```python
from build123d import *

# Parameters (mm, degrees)
F1_DEPTH = 50.8
F3_DEPTH = 50.801
F4_R     = 9.525
F5_DEPTH = 50.801
F6_R     = 63.5
F6_W     = 50.8
F6_H     = 50.8
F7_DEPTH = 12.7
F8_R     = 3.81


with BuildPart() as f1:
    # F0 (on Front) → F1 (new body)
    with BuildSketch(Plane.XZ):
        Polygon((-38.3064501607, 0), (-38.3064501607, 59.24468064), (-51.0064501607, 59.24468064), (-51.0064501607, -16.95531936), (-0.2064501607, -16.95531936), (-0.2064501607, 59.24468064), (-12.9064501607, 59.24468064), (-12.9064501607, 0), align=None)
    extrude(amount=F1_DEPTH)

    # F2 (on face) → F3 (cut, through all)
    with BuildSketch(Plane.YZ.offset(-0.2064501607)):
        with BuildLine():
            ThreePointArc((-50.8, 33.84468064), (-43.3605122421, 51.8051928821), (-25.4, 59.24468064))
            Line((-25.4, 59.24468064), (-50.8, 59.24468064))
            Line((-50.8, 59.24468064), (-50.8, 33.84468064))
        make_face()
        with BuildLine():
            ThreePointArc((-25.4, 59.24468064), (-7.4394877579, 51.8051928821), (0, 33.84468064))
            Line((0, 33.84468064), (0, 59.24468064))
            Line((0, 59.24468064), (-25.4, 59.24468064))
        make_face()
    extrude(amount=-F3_DEPTH, mode=Mode.SUBTRACT)

    # F4 (on face) → F5 (cut, through all)
    with BuildSketch(Plane.YZ.offset(-0.2064501607)):
        with Locations((-25.4, 33.84468064)):
            Circle(F4_R)
    extrude(amount=-F5_DEPTH, mode=Mode.SUBTRACT)

    # F6 (on face) → F7 (join)
    with BuildSketch(Plane(origin=(0, 0, -16.95531936), x_dir=(1, 0, 0), z_dir=(0, 0, -1))):
        with Locations((-25.6064501607, 25.4)):
            Circle(F6_R)
        with BuildLine():
            ThreePointArc((-19.2726698552, 69.3964285714), (5.824446263, 56.8308964237), (18.3899784107, 31.7337803056))
            ThreePointArc((18.3899784107, 31.7337803056), (23.1703455028, 30.0477240974), (25.1935498393, 25.4))
            ThreePointArc((25.1935498393, 25.4), (23.1703455028, 20.7522759026), (18.3899784107, 19.0662196944))
            ThreePointArc((18.3899784107, 19.0662196944), (5.824446263, -6.0308964237), (-19.2726698552, -18.5964285714))
            ThreePointArc((-19.2726698552, -18.5964285714), (-19.2605063799, -18.8230693282), (-19.2564501607, -19.05))
            ThreePointArc((-19.2564501607, -19.05), (-25.8333808326, -25.3959437809), (-31.9402304663, -18.5964285714))
            ThreePointArc((-31.9402304663, -18.5964285714), (-57.0373465845, -6.0308964237), (-69.6028787322, 19.0662196944))
            ThreePointArc((-69.6028787322, 19.0662196944), (-76.4064501607, 25.4), (-69.6028787322, 31.7337803056))
            ThreePointArc((-69.6028787322, 31.7337803056), (-57.0373465845, 56.8308964237), (-31.9402304663, 69.3964285714))
            ThreePointArc((-31.9402304663, 69.3964285714), (-25.8333808326, 76.1959437809), (-19.2564501607, 69.85))
            ThreePointArc((-19.2564501607, 69.85), (-19.2605063799, 69.6230693282), (-19.2726698552, 69.3964285714))
        make_face(mode=Mode.SUBTRACT)
        with BuildLine():
            ThreePointArc((18.3899784107, 19.0662196944), (12.4935498393, 25.4), (18.3899784107, 31.7337803056))
            ThreePointArc((18.3899784107, 31.7337803056), (5.824446263, 56.8308964237), (-19.2726698552, 69.3964285714))
            ThreePointArc((-19.2726698552, 69.3964285714), (-25.6064501607, 63.5), (-31.9402304663, 69.3964285714))
            ThreePointArc((-31.9402304663, 69.3964285714), (-57.0373465845, 56.8308964237), (-69.6028787322, 31.7337803056))
            ThreePointArc((-69.6028787322, 31.7337803056), (-65.4087260633, 29.7267956636), (-63.7064501607, 25.4))
            ThreePointArc((-63.7064501607, 25.4), (-65.4087260633, 21.0732043364), (-69.6028787322, 19.0662196944))
            ThreePointArc((-69.6028787322, 19.0662196944), (-57.0373465845, -6.0308964237), (-31.9402304663, -18.5964285714))
            ThreePointArc((-31.9402304663, -18.5964285714), (-25.6064501607, -12.7), (-19.2726698552, -18.5964285714))
            ThreePointArc((-19.2726698552, -18.5964285714), (5.824446263, -6.0308964237), (18.3899784107, 19.0662196944))
        make_face()
        with Locations((-25.6064501607, 25.4)):
            Rectangle(F6_W, F6_H, mode=Mode.SUBTRACT)
        with Locations((-25.6064501607, 25.4)):
            Rectangle(F6_W, F6_H)
    extrude(amount=F7_DEPTH)

    # F8
    f8_edges = [f1.edges().sort_by_distance(p)[0] for p in [
        (-51.00645, -25.4, -16.955319),
        (-25.60645, -50.8, -16.955319),
        (-0.20645, -25.4, -16.955319),
        (-25.60645, 0, -16.955319),
        (-89.10645, -25.4, -16.955319),
    ]]
    fillet(f8_edges, radius=F8_R)


solid = f1.part
```
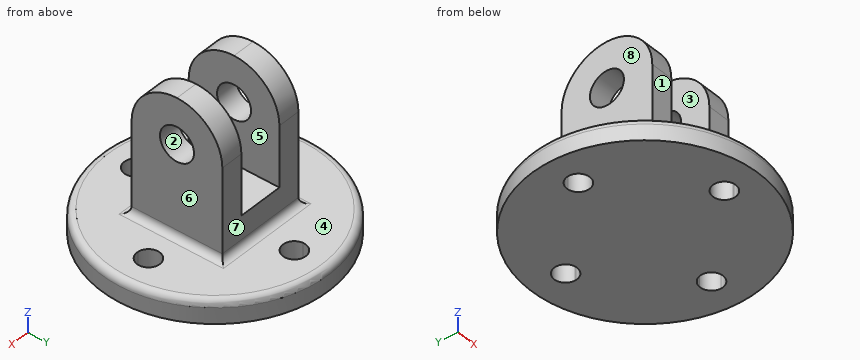
CAD build for the part. Positions are in the model's coordinates, mm. Face numbers are marked on the shaded views. A direction names the side the tool comes from. Round coordinates to 2 decimals unless told otherwise and drop trailing zeros. Order: outer loops, then holes, each group sorted by start corner. A loop starts at its lowest first (then second) coordinate and runs counter-clockwise, first axis right, second up. Notation, with made-up numbers: (16.25, 46.25) - (23.25, 46.25) arc R24 cw to (23.25, 82.25) - close; hole circle Ø3 at (68, 10.5). An arc over 180 degrees is marked (long way). Use CSV: the item, a comma, the result in double quotes. Start each with the question number.
1) Wall check: L1, parallel to X at y = -40.5, z = 44; L2, parallel to Z at x = -8, y = -25; L3, parallel to Y at x = -40, z = 29. Give the ranges that are in metal, low to high. Write a range as [from, to].
2) Saw through at B-B (z = 18). List the corners of the cut face in (x, y), and give its area (3 significant figures).
3) Pin check, flat tips, straight feed: pin 1 Ø5 at (y, z) = (-9, 35) entering from +X; pin 2 Ø14 at (x, z) = (-36, 18.5) entering from -Y; pin 3 Ø3 at (x, z) = (-41, 48.5) entering from +Y. Stop position of each tip, or through.
4) Saw through at A-A (z = -23). List the corners of the cut face in (x, y).
5) Saw through at C-C (z = -7). List the corners of the cut face in (x, y).
6) Tool access for the marked faces 4, 5, 6, 7 and 8: list every direction of +Z, -Z, +X, -X, +Y, -Y with a clear straight run to the whole face (end or side of a thin tool).
7) Two-plate mould, pull along Y, no slides. Class the marked faces 1, 2 and 3: pulls with the +Y half, pulls with the -Y half, needs draft (parallel to the pull), parting line crosses it, or undercut.
Values follow:
1,L1,"x = [-51.01, -38.31], [-12.91, -0.21]"
1,L2,"z = [-29.66, 24.33], [43.36, 59.24]"
1,L3,"y = [-50.8, -33.6], [-17.2, 0]"
2,outline,"(-51.01, -50.8) - (-38.31, -50.8) - (-38.31, 0) - (-51.01, 0) - close; (-12.91, -50.8) - (-0.21, -50.8) - (-0.21, 0) - (-12.91, 0) - close"
2,area,"1,290 mm2"
3,pin 1,"stops at x = -0.21"
3,pin 2,"stops at y = -50.8"
3,pin 3,"stops at y = -3.67"
4,outline,"circle Ø127 at (-25.61, -25.4); hole circle Ø12.7 at (-70.06, -25.4); hole circle Ø12.7 at (-25.61, -69.85); hole circle Ø12.7 at (-25.61, 19.05); hole circle Ø12.7 at (18.84, -25.4)"
5,outline,"(-51.01, -50.8) - (-0.21, -50.8) - (-0.21, 0) - (-51.01, 0) - close"
6,face 4,"+Z"
6,face 5,"+Z, +Y, -Y"
6,face 6,"+Z, +X, +Y, -Y"
6,face 7,"+Z, +X, -X, +Y"
6,face 8,"+Z, -X, +Y, -Y"
7,face 1,"pulls with the -Y half"
7,face 2,"undercut"
7,face 3,"needs draft"
